For this review, take the finished solid that the model builds, in its own axes (mm). Face numbers are marked on the shaded views. Round coordinates to 2 decimals unless told otherwise and drop trailing zeros. Order: outer loops, then holes, each group sorted by start corner. A loop starts at its lowest first (then second) coordinate and runs counter-clockwise, first axis right, second up.
```python
from build123d import *

# Parameters (mm, degrees)
F0_R     = 76.2
F3_T     = -6.35
F0_R_2   = 95.25
F4_DEPTH = 6.35


with BuildPart() as f2:
    # F2: sweep along a path in F1
    with BuildLine(Plane.XY) as f2_path:
        Line((0, 0), (0, 152.4))
        ThreePointArc((0, 152.4), (44.6369265472, 260.1630734528), (152.4, 304.8))
        Line((152.4, 304.8), (304.8, 304.8))
    # F0 (on Front) → F2 (sweep)
    with BuildSketch(Plane.XZ):
        Circle(F0_R)
    sweep(path=f2_path.line)

    # F3
    f3_openings = [f2.faces().sort_by_distance(p)[0] for p in [
        (0, 0, 0),
        (304.8, 304.8, 0),
    ]]
    offset(amount=F3_T, openings=f3_openings)

    # F0 (on Front) → F4 (join)
    with BuildSketch(Plane.XZ):
        Circle(F0_R_2)
        Circle(F0_R, mode=Mode.SUBTRACT)
    extrude(amount=-F4_DEPTH)


solid = f2.part
```
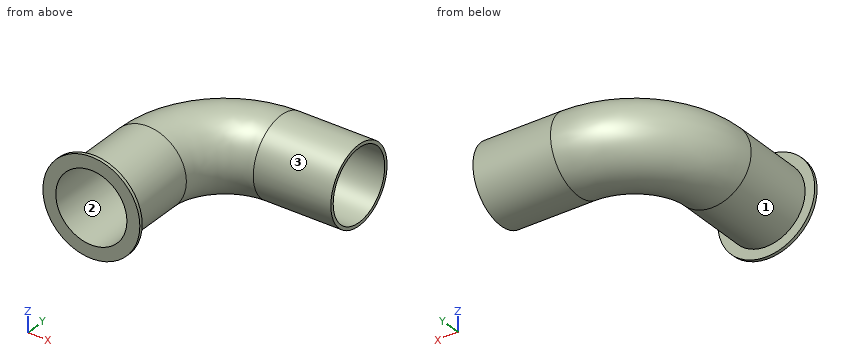
Q1. Mouldability with a two-part tool opening along Y and no side actions: class the marked faces 1, 2 and 3 as +Y half, -Y half, draft (parallel to the pull), parting line (faces both ways), or undercut.
Q2. Take a section at B-B, the plane x = 278. State the section outline as (y, z) points, plus the area to 3 significant figures.
Q3. Take a section at A-A, the plane z = -22. State the section outline as (x, y) points, plus the area to 3 significant figures.
Q4. Clearance check with flat-ended pins moving along their axes: pin 1 (12 mm diameter, centred on x = 22.5, y = 63, fed in from -Z); pin 2 (8 mm diameter, centred on y = 54.5, z = 53.5, fed in from +X); pin 3 (1.5 mm diameter, centred on x = 209.5, y = 337, fed in from +Z). State where each tip first meets the part, or that it passes through.
Q5. Wall thickness on line 1 (Y direction, x = 229, z = -2.5); line 2 (X direction, y = 40, z = 42); line 3 (Z direction, x = 0, y = 70): over which ranges is each line inside the solid? List them lowest first.
Working result:
1. face 1: undercut
1. face 2: draft
1. face 3: parting line
2. outline: circle Ø152.4 at (304.8, 0); hole circle Ø139.7 at (304.8, 0)
2. area: 2,910 mm2
3. outline: (-92.67, 0) - (-66.29, 0) - (-66.29, 152.4) arc R218.69 cw to (152.4, 371.09) - (304.8, 371.09) - (304.8, 377.76) - (152.4, 377.76) arc R225.36 ccw to (-72.96, 152.4) - (-72.96, 6.35) - (-92.67, 6.35) - close; (66.29, 0) - (92.67, 0) - (92.67, 6.35) - (72.96, 6.35) - (72.96, 152.4) arc R79.44 cw to (152.4, 231.84) - (304.8, 231.84) - (304.8, 238.51) - (152.4, 238.51) arc R86.11 ccw to (66.29, 152.4) - close
3. area: 7,500 mm2
4. pin 1: stops at z = -74.39
4. pin 2: stops at x = 57.93
4. pin 3: stops at z = 69.41
5. line 1: y = 228.64 to 234.99, 374.61 to 380.96
5. line 2: x = -63.58 to -55.81, 55.81 to 63.58
5. line 3: z = -76.2 to -69.85, 69.85 to 76.2
